Design review of the part built by this model. Coordinates are the model's own, in mm. A direction names the side the tool comes from. Round coordinates to 2 decimals unless told otherwise and drop trailing zeros. Loops run counter-clockwise (first coordinate to the right, second up) from the corner with the lowest first, then second, coordinate; pieces in that order, holes last. Notation, with made-up numbers: (44.25, 42) -> (71.25, 42) arc R24 ccw to (71.25, 56) -> close; hole circle Ø4 at (84, 47.5). An arc over 180 degrees is marked (long way). Answer as CSV lines item,"result". Start each with the question number.
(1) Take a section at D-D, the plane x = 21. Write out the cut boundary in (y, z).
(2) To check wall thickness, follow line 1 (Y direction, x = 15.5, z = 0); line 2 (Y direction, x = 4.5, z = 0); line 3 (Y direction, x = 31.75, z = 0). State the ranges of each line that lie inside material, in increasing order. Write a range as from..to.
(3) Draft analysis for pull direction Z (two halves, no side actions). For faces 4 (the face through (4.437, 22.804, -2.994)), 5 (the face through (31.888, -16.856, -8.767)), 6 (the face through (24, 18, 7)), state which applies: +Z half, -Z half, draft (parallel to the pull), parting line (faces both ways), or undercut.
(4) For P1, Ø4, axis at y = 1, z = -33, coming from the -X side; P2, Ø5, axis at x = 11.5, z = 7.5, coming from the +Y side; P3, Ø3.5, axis at x = 26, y = 12.5, coming from the -Z side, all flat-tipped, find the tip position at first contact; note any pin that passes through.
(5) Machinability: for faces 1 (the face through (18.93, -21.477, 4.769)), 2 (the face through (5.916, 37.966, -0.521)), 3 (the face through (26, 12, -2.5)), which of the approach directions +Z, -Z, +X, -X, +Y, -Y give a long, thin tool a straight path to every point of the face, cutting with its end or side? Answer none if there is none.
(6) Take a section at B-B, the plane x = 6.5. Write out the cut boundary in (y, z).
from build123d import *

# Parameters (mm, degrees)
SKETCH_1_R          = 45
EXTRUDE_1_DEPTH     = 14
SKETCH_2_R          = 22
EXTRUDE_2_DEPTH     = 10
SKETCH_3_R          = 19
EXTRUDE_3_DEPTH     = 16
SKETCH_4_R          = 23
CUT_EXTRUDE_1_DEPTH = 12
SKETCH_5_R          = 11
CUT_EXTRUDE_2_DEPTH = 29
SKETCH_6_W          = 28
SKETCH_6_H          = 14
CUT_EXTRUDE_3_DEPTH = 2.5
SKETCH_7_R          = 4
CUT_EXTRUDE_4_DEPTH = 12
FILLET_1_R          = 3


with BuildPart() as part:
    # 草图1 → 凸台-拉伸1 (new body)
    with BuildSketch(Plane(origin=(0, 0, 0), x_dir=(0, 0, -1), z_dir=(1, 0, 0))):
        Circle(SKETCH_1_R)
    extrude(amount=EXTRUDE_1_DEPTH)

    # 草图2 → 凸台-拉伸2 (add)
    with BuildSketch(Plane(origin=(14, 0, 0), x_dir=(0, 0, -1), z_dir=(1, 0, 0))):
        Circle(SKETCH_2_R)
    extrude(amount=EXTRUDE_2_DEPTH)

    # 草图3 → 凸台-拉伸3 (add)
    with BuildSketch(Plane(origin=(24, 0, 0), x_dir=(0, 0, -1), z_dir=(1, 0, 0))):
        Circle(SKETCH_3_R)
    extrude(amount=EXTRUDE_3_DEPTH)

    # 草图4 → 切除-拉伸1 (cut)
    with BuildSketch(Plane.ZY):
        Circle(SKETCH_4_R)
    extrude(amount=-CUT_EXTRUDE_1_DEPTH, mode=Mode.SUBTRACT)

    # 草图5 → 切除-拉伸2 (cut, through all)
    with BuildSketch(Plane.ZY.offset(-12)):
        Circle(SKETCH_5_R)
    extrude(amount=-CUT_EXTRUDE_2_DEPTH, mode=Mode.SUBTRACT)

    # 草图6 → 切除-拉伸3 (cut, symmetric)
    with BuildSketch(Plane.XY):
        with Locations((26, 7)):
            Rectangle(SKETCH_6_W, SKETCH_6_H)
    extrude(amount=CUT_EXTRUDE_3_DEPTH, both=True, mode=Mode.SUBTRACT)

    # 草图7 → 切除-拉伸4 (cut)
    with BuildSketch(Plane.ZY):
        with Locations((0, 34)):
            Circle(SKETCH_7_R)
        with Locations((34, 0)):
            Circle(SKETCH_7_R)
        with Locations((0, -34)):
            Circle(SKETCH_7_R)
        with BuildLine():
            ThreePointArc((-38, 0), (-34, -4), (-30, 0))
            Line((-30, 0), (-38, 0))
        make_face()
        with BuildLine():
            Line((-38, 0), (-30, 0))
            ThreePointArc((-30, 0), (-34, 4), (-38, 0))
        make_face()
    extrude(amount=-CUT_EXTRUDE_4_DEPTH, mode=Mode.SUBTRACT)

    # 圆角1
    fillet_1_edges = [part.edges().sort_by_distance(p)[0] for p in [
        (12, 0, -23),
    ]]
    fillet(fillet_1_edges, radius=FILLET_1_R)


solid = part.part
The answers:
1,outline,"circle Ø44 at (0, 0); hole (10.71, -2.5) -> (14, -2.5) -> (14, 2.5) -> (10.71, 2.5) arc R11 ccw (long way) to start"
2,line 1,"-22..-11, 14..22"
2,line 2,"-45..-38, -30..-23, 23..30, 38..45"
2,line 3,"-19..-11, 14..19"
3,face 4,"undercut"
3,face 5,"parting line"
3,face 6,"draft"
4,P1,"x = 12"
4,P2,"y = 44.72"
4,P3,"z = -15.67"
5,face 1,"+X"
5,face 2,"-X"
5,face 3,"+X, -X"
6,outline,"circle Ø90 at (0, 0); hole circle Ø8 at (-34, 0); hole circle Ø46 at (0, 0); hole circle Ø8 at (0, -34); hole circle Ø8 at (0, 34); hole circle Ø8 at (34, 0)"
